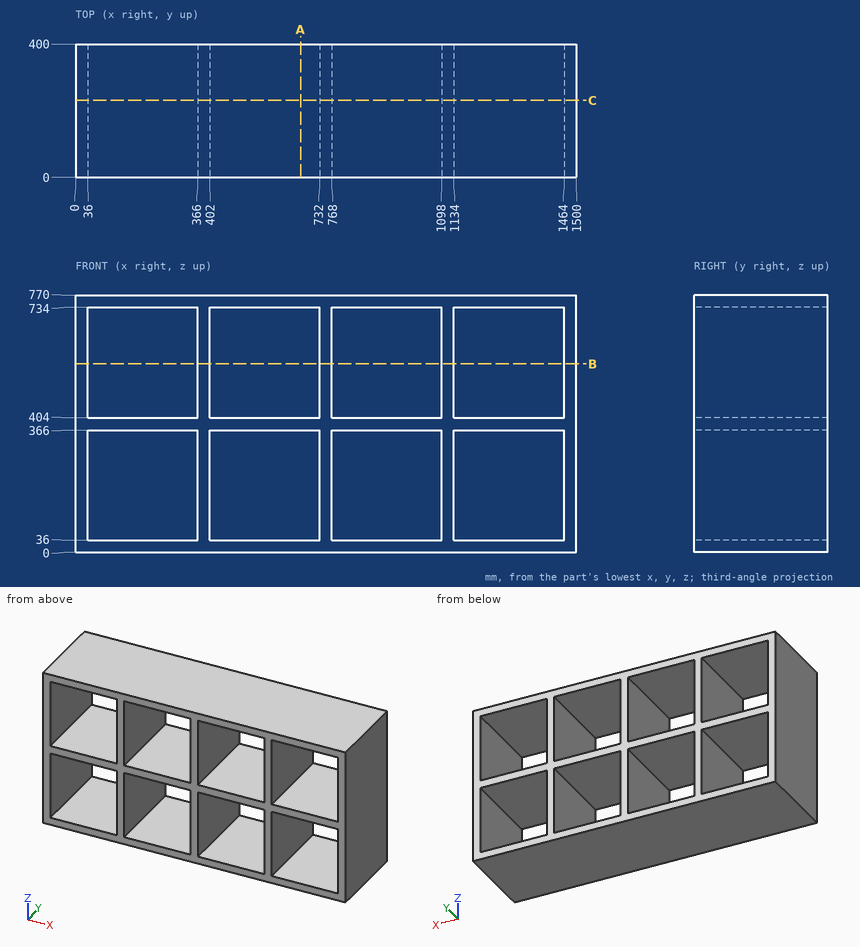
Could you check a few things on this drawing? It's one solid part, dimensions in mm from its lowest x, y, z. Coordinates: 2 decimals unless noted, no trailing zeros. Order: outer loops, then holes, each group sorted by start corner. A loop starts at its lowest first (then second) coordinate and runs counter-clockwise, first axis right, second up.
1. If we section it at B-B (z = 565): Please give me the cut outline in (x, y).
2. I need wall thicknesses on line 1 (Z direction, x = 1301.5, y = 316); line 2 (X direction, y = 140, z = 443.5). Which ranges of each line are inside material? Lowest first, please.
3. If we section it at C-C (y = 231): Give the number of separate pieces and of enclosed holes in the cut face, then the cut area to 3 significant figures.
4. If we section it at A-A (x = 674.5): Please give me the cut outline in (y, z), then the cut area to 3 significant figures.
Entries:
1. outline: (0, 0) - (36, 0) - (36, 400) - (0, 400) - close; (366, 0) - (402, 0) - (402, 400) - (366, 400) - close; (732, 0) - (768, 0) - (768, 400) - (732, 400) - close; (1098, 0) - (1134, 0) - (1134, 400) - (1098, 400) - close; (1464, 0) - (1500, 0) - (1500, 400) - (1464, 400) - close
2. line 1: z = 0 to 36, 366 to 404, 734 to 770
2. line 2: x = 0 to 36, 366 to 402, 732 to 768, 1098 to 1134, 1464 to 1500
3. separate pieces: 1
3. enclosed holes: 8
3. area: 284,000 mm2
4. outline: (0, 0) - (400, 0) - (400, 36) - (0, 36) - close; (0, 366) - (400, 366) - (400, 404) - (0, 404) - close; (0, 734) - (400, 734) - (400, 770) - (0, 770) - close
4. area: 44,000 mm2
